Part model, mm, in its own coordinate system. A direction names the side the tool comes from. Round coordinates to 2 decimals unless told otherwise and drop trailing zeros. Loops run counter-clockwise (first coordinate to the right, second up) from the corner with the lowest first, then second, coordinate; pieces in that order, holes last. Notation, with made-up numbers: M 73.5,27 L 78.5,27 A15 cw 78.5,45 Z; hole C 47,79 d4. An arc over 180 degrees is marked long. Put each result on its own line as item: value. Start each with the question number.
1) Pull direction X, two halves, no side cores. Call faces 5 (the flat face through (-33.364, -39.021, 0.301)), 6 (the flat face through (-8.365, -14.022, 0.301)), 7 (the flat face through (-28, -54.39, -16)), 8 (the flat face through (32.5, -52, -1)): +X half, -X half, draft (parallel to the pull), parting line (faces both ways), or undercut.
2) Drop flat-ended pins along their axis: pin 1 Ø3 at (x, y) = (19.5, -51.5) entering from +Z; pin 2 Ø1.5 at (x, z) = (6, -3.5) entering from +Y; pin 3 Ø6.5 at (y, z) = (-52.5, 2.5) entering from +X. Give the stop position or say it passes through.
3) Slice it at B-B on y = -33. Give the cut face in (x, z), then the cut area to 3 significant figures.
4) Which spindle directions (+Z, -Z, +X, -X, +Y, -Y) get a long thin tool onto all of the face, cutting with end or side? Do faces 1 (the flat face through (-39, -42, 0)), 2 (the flat face through (-19, -51, 12.35)), 3 (the flat face through (-28, -52, -17.15)), 4 (the flat face through (31, -49.39, -16)). Say none if no direction does.
5) Slice it at D-D on z = -12. Give the cut face in (x, y), then the cut area to 3 significant figures.
6) Slice it at A-A on z = 11. Give the cut face in (x, y), then the cut area to 3 significant figures.
7) Slice it at C-C on x = -14. Give the cut face in (y, z).
8) Probe line 1 along Y through (x, z) = (0, 20); line 2 along X through (y, z) = (-47, -9); line 3 along Z through (x, y) = (27, -50). List the from-to ranges inside material, lowest first.
```python
from build123d import *

# Parameters (mm, degrees)
BOSS_EXTRUDE1_DEPTH  = 21.5
BOSS_EXTRUDE7_START  = 5
SKETCH11_R           = 5.85
BOSS_EXTRUDE7_DEPTH  = 10
SKETCH12_R           = 2.85
CUT_EXTRUDE3_DEPTH   = 9
BOSS_EXTRUDE8_START  = 0.1
SKETCH14_W           = 5
SKETCH14_H           = 43
BOSS_EXTRUDE8_DEPTH  = 18.432718
SKETCH17_W           = 9.4
SKETCH17_H           = 2.3
BOSS_EXTRUDE10_DEPTH = 5
SKETCH18_W           = 8.15
SKETCH18_H           = 14.45
BOSS_EXTRUDE11_DEPTH = 1


with BuildPart() as part:
    # Sketch1 → Boss-Extrude1 (new body, symmetric)
    with BuildSketch(Plane.XY):
        Polygon((0, 0), (-42, -42), (-36.343145751, -42), (-32.343145751, -38), (-20.5, -26.156854249), (-16.5, -25.156854249), (16.5, -25.156854249), (20.5, -26.156854249), (32.343145751, -38), (36.343145751, -42), (42, -42), align=None)
        Polygon((-16.5, -22.156854249), (0, -5.656854249), (16.5, -22.156854249), align=None, mode=Mode.SUBTRACT)
    extrude(amount=BOSS_EXTRUDE1_DEPTH, both=True)

    # Sketch11 → Boss-Extrude7 (add)
    with BuildSketch(Plane.XY.offset(21.5).offset(BOSS_EXTRUDE7_START)):
        with Locations((0, -23.656854249)):
            Circle(SKETCH11_R)
    extrude(amount=-BOSS_EXTRUDE7_DEPTH)

    # Sketch12 → Cut-Extrude3 (cut)
    with BuildSketch(Plane(origin=(0, 0, 26.5), x_dir=(-1, 0, 0), z_dir=(0, 0, -1))):
        with Locations((0, -23.656854249)):
            Circle(SKETCH12_R)
    extrude(amount=CUT_EXTRUDE3_DEPTH, mode=Mode.SUBTRACT)

    # Sketch14 → Boss-Extrude8 (add)
    with BuildSketch(Plane(origin=(0, -49.48957189, 0), x_dir=(1, 0, 0), z_dir=(0, 1, 0)).offset(BOSS_EXTRUDE8_START)):
        with Locations((-27.8, 0)):
            Rectangle(SKETCH14_W, SKETCH14_H)
    boss_extrude8 = extrude(amount=BOSS_EXTRUDE8_DEPTH)

    # Sketch17 → Boss-Extrude10 (add)
    with BuildSketch(Plane.XZ.offset(49.38957189)):
        Polygon((-17.15, 12.35), (-17.15, -2.1), (-32.5, -2.1), (-32.5, 0.2), (-19.45, 0.2), (-19.45, 12.35), align=None)
        with Locations((-27.8, -16)):
            Rectangle(SKETCH17_W, SKETCH17_H)
    boss_extrude10 = extrude(amount=BOSS_EXTRUDE10_DEPTH)

    # Sketch18 → Boss-Extrude11 (add)
    with BuildSketch(Plane(origin=(0, -49.38957189, 0), x_dir=(1, 0, 0), z_dir=(0, 1, 0))):
        with Locations((-21.225, -5.125)):
            Rectangle(SKETCH18_W, SKETCH18_H)
    boss_extrude11 = extrude(amount=BOSS_EXTRUDE11_DEPTH)

    # Mirror2: Boss-Extrude8, Boss-Extrude10, Boss-Extrude11 across plane
    add(boss_extrude8.mirror(Plane(origin=(0, 0, 0), x_dir=(0, 0, 1), z_dir=(1, 0, 0))))
    add(boss_extrude10.mirror(Plane(origin=(0, 0, 0), x_dir=(0, 0, 1), z_dir=(1, 0, 0))))
    add(boss_extrude11.mirror(Plane(origin=(0, 0, 0), x_dir=(0, 0, 1), z_dir=(1, 0, 0))))

    # Sketch15 → Revolve1 (revolve)
    with BuildSketch(Plane(origin=(0, 0, 0), x_dir=(0, 0, -1), z_dir=(1, 0, 0))):
        Polygon((-16.5, -17.806854249), (-10.65, -23.656854249), (-16.5, -23.656854249), align=None)
    revolve(axis=Axis((0, -23.656854249, 10.65), (0, 0, 1)))


solid = part.part
```
Recorded:
1. face 5: undercut
1. face 6: undercut
1. face 7: draft
1. face 8: +X half
2. pin 1: stops at z = 12.35
2. pin 2: stops at y = -5.25
2. pin 3: stops at x = 32.5
3. outline: M -33,-21.5 L -25.3,-21.5 L -25.3,21.5 L -33,21.5 Z; M 25.3,-21.5 L 33,-21.5 L 33,21.5 L 25.3,21.5 Z
3. area: 662 mm2
4. face 1: +Z, -Z, -X, -Y
4. face 2: +Z, -Y
4. face 3: -Z, +X, -X, -Y
4. face 4: +Z, -Z, +X
5. outline: M -42,-42 L -36.34,-42 L -30.3,-35.96 L -30.3,-49.39 L -25.3,-49.39 L -25.3,-30.96 L -20.5,-26.16 L -16.5,-25.16 L 16.5,-25.16 L 20.5,-26.16 L 25.3,-30.96 L 25.3,-49.39 L 30.3,-49.39 L 30.3,-35.96 L 36.34,-42 L 42,-42 L 0,0 Z; hole M -16.5,-22.16 L 16.5,-22.16 L 0,-5.66 Z
5. area: 714 mm2
6. outline: M -42,-42 L -36.34,-42 L -30.3,-35.96 L -30.3,-49.39 L -19.45,-49.39 L -19.45,-54.39 L -17.15,-54.39 L -17.15,-48.39 L -25.3,-48.39 L -25.3,-30.96 L -20.5,-26.16 L -16.5,-25.16 L 16.5,-25.16 L 20.5,-26.16 L 25.3,-30.96 L 25.3,-48.39 L 17.15,-48.39 L 17.15,-54.39 L 19.45,-54.39 L 19.45,-49.39 L 30.3,-49.39 L 30.3,-35.96 L 36.34,-42 L 42,-42 L 0,0 Z; hole M -16.5,-22.16 L 16.5,-22.16 L 0,-5.66 Z
6. area: 753 mm2
7. outline: M -25.16,-21.5 L -22.16,-21.5 L -22.16,21.5 L -25.16,21.5 Z; M -19.66,-21.5 L -14,-21.5 L -14,21.5 L -19.66,21.5 Z
8. line 1: y = -29.51 to -26.51, -20.81 to -17.81, -5.66 to 0
8. line 2: x = -30.3 to -25.3, 25.3 to 30.3
8. line 3: z = -17.15 to -14.85, -2.1 to 0.2
